Design review of the part built by this model. Coordinates are the model's own, in mm. Face numbers are marked on the shaded views. A direction names the side the tool comes from. Give positions to 0.01 mm unless a question says otherwise; leave off trailing zeros. Order: outer loops, then holes, each group sorted by start corner. A loop starts at its lowest first (then second) coordinate and runs counter-clockwise, first axis right, second up. Notation, with made-up numbers: (68.5, 3) -> (88.5, 3) arc R15 ccw to (88.5, 7) -> close; hole circle Ø4 at (40, 76). An arc over 180 degrees is marked (long way). Return JSON: item names as keys, results as strings.
```python
from build123d import *

# Parameters (mm, degrees)
SKETCH1_W           = 66
SKETCH1_H           = 48
BOSS_EXTRUDE1_DEPTH = 5
SKETCH2_W           = 10
SKETCH2_H           = 10
BOSS_EXTRUDE2_DEPTH = 44
SKETCH3_R           = 1
CUT_EXTRUDE1_DEPTH  = 7
SKETCH4_W           = 66
SKETCH4_H           = 70
BOSS_EXTRUDE3_DEPTH = 3
BOSS_EXTRUDE4_DEPTH = 3
SKETCH6_R           = 1
CUT_EXTRUDE2_DEPTH  = 3


with BuildPart() as part:
    # Sketch1 → Boss-Extrude1 (new body)
    with BuildSketch(Plane(origin=(0, 0, 0), x_dir=(1, 0, 0), z_dir=(0, 1, 0))):
        Rectangle(SKETCH1_W, SKETCH1_H)
    extrude(amount=BOSS_EXTRUDE1_DEPTH)

    # Sketch2 → Boss-Extrude2 (add)
    with BuildSketch(Plane(origin=(0, 5, 0), x_dir=(1, 0, 0), z_dir=(0, 1, 0))):
        with Locations((7, 19)):
            Rectangle(SKETCH2_W, SKETCH2_H)
        with Locations((7, -19)):
            Rectangle(SKETCH2_W, SKETCH2_H)
    extrude(amount=BOSS_EXTRUDE2_DEPTH)

    # Sketch3 → Cut-Extrude1 (cut)
    with BuildSketch(Plane(origin=(0, 49, 0), x_dir=(1, 0, 0), z_dir=(0, 1, 0))):
        with Locations(Location((7, 19, 0), (0, 0, 270))):
            Circle(SKETCH3_R)
        with Locations(Location((7, -19, 0), (0, 0, 270))):
            Circle(SKETCH3_R)
    extrude(amount=-CUT_EXTRUDE1_DEPTH, mode=Mode.SUBTRACT)

    # Sketch4 → Boss-Extrude3 (add)
    with BuildSketch(Plane.XZ):
        Rectangle(SKETCH4_W, SKETCH4_H)
    extrude(amount=BOSS_EXTRUDE3_DEPTH)

    # Sketch5 → Boss-Extrude4 (add)
    with BuildSketch(Plane(origin=(33, 0, 0), x_dir=(0, 0, -1), z_dir=(1, 0, 0))):
        Polygon((-24, 5), (-35, 0), (-24, 0), align=None)
        Polygon((24, 5), (24, 0), (35, 0), align=None)
    boss_extrude4 = extrude(amount=-BOSS_EXTRUDE4_DEPTH)

    # Mirror1: Boss-Extrude4 across plane
    add(boss_extrude4.mirror(Plane(origin=(0, 0, 0), x_dir=(0, 0, 1), z_dir=(1, 0, 0))))

    # Sketch6 → Cut-Extrude2 (cut)
    with BuildSketch(Plane(origin=(0, 0, 0), x_dir=(1, 0, 0), z_dir=(0, 1, 0))):
        with Locations(Location((-22, 29.5, 0), (0, 0, 270))):
            Circle(SKETCH6_R)
        with Locations(Location((22, 29.5, 0), (0, 0, 270))):
            Circle(SKETCH6_R)
    cut_extrude2 = extrude(amount=-CUT_EXTRUDE2_DEPTH, mode=Mode.SUBTRACT)

    # Mirror2: Cut-Extrude2 across plane
    add(cut_extrude2.mirror(Plane.XY), mode=Mode.SUBTRACT)


solid = part.part
```
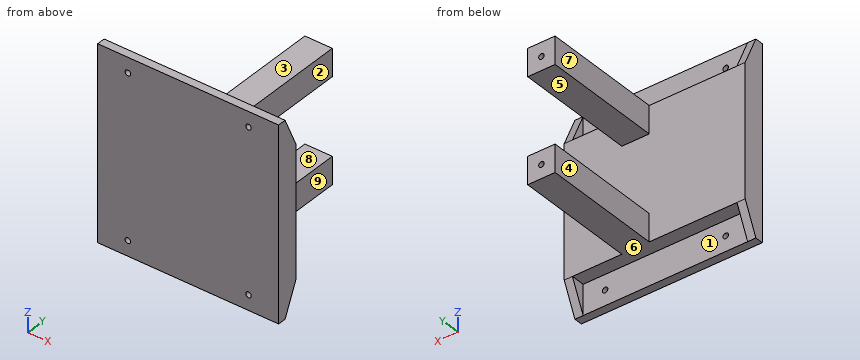
Item 1: Add section B-B (y = 34.5). Give the boundary of the cut face in (x, z), plus the area to 3 significant figures.
Result set:
{"outline": "(2, -24) -> (12, -24) -> (12, -14) -> (2, -14) -> close; (2, 14) -> (12, 14) -> (12, 24) -> (2, 24) -> close", "area": "200 mm^2"}
Item 2: Machinability: for the marked faces 1, 2, 3, 4 and 5, which of the approach directions +Z, -Z, +X, -X, +Y, -Y give a long, thin tool a straight path to every point of the face, cutting with its end or side? Answer none if there is none.
Result set:
{"face 1": "-Z, +Y", "face 2": "+Z, -Z, +X, +Y", "face 3": "+Z, +Y", "face 4": "+Z, -Z, -X, +Y", "face 5": "+X, -X, +Y"}
Item 3: Mouldability with a two-part tool opening along X and no side actions: class the marked faces 6, 7, 8 and 9 as released by +X, released by -X, zero draft, split by the parting line, or undercut.
Result set:
{"face 6": "undercut", "face 7": "released by -X", "face 8": "zero draft", "face 9": "released by +X"}
Item 4: Add section C-C (x = 22). Give the boundary of the cut face in (y, z).
Result set:
{"outline": "(-3, -35) -> (0, -35) -> (0, -30.5) -> (-3, -30.5) -> close; (-3, -28.5) -> (0, -28.5) -> (0, -24) -> (5, -24) -> (5, 24) -> (0, 24) -> (0, 28.5) -> (-3, 28.5) -> close; (-3, 30.5) -> (0, 30.5) -> (0, 35) -> (-3, 35) -> close"}
Item 5: Add section A-A (z = 29.5). Give the boundary of the cut face in (x, y), plus the area to 3 significant figures.
Result set:
{"outline": "(-33, -3) -> (-23, -3) -> (-23, 0) -> (-30, 0) -> (-30, 2.5) -> (-33, 2.5) -> close; (-21, -3) -> (21, -3) -> (21, 0) -> (-21, 0) -> close; (23, -3) -> (33, -3) -> (33, 2.5) -> (30, 2.5) -> (30, 0) -> (23, 0) -> close", "area": "201 mm^2"}
Item 6: For pin 1 (8 mm diameter, centred on x = 5.5, y = 18.5, fed in from +Z); pin 2 (5 mm diameter, centred on y = 27.5, z = 19, fed in from -X); pin 3 (0.6 mm diameter, centred on x = 7, z = 19, fed in from +Y), all flat-tipped, find the tip position at first contact; note any pin that passes through.
Result set:
{"pin 1": "stops at z = 24", "pin 2": "stops at x = 2", "pin 3": "stops at y = 42"}
Item 7: Wall thickness on L1, parallel to X at y = -1.75, z = 29.5; L2, parallel to Z at x = 4.5, y = 44; L3, parallel to Y at x = 18, z = -12.5: over which ranges is each line inside the solid? List them lowest first. Write a range as [from, to].
Result set:
{"L1": "x = [-33, -23], [-21, 21], [23, 33]", "L2": "z = [-24, -14], [14, 24]", "L3": "y = [-3, 5]"}
Item 8: Add section D-D (x = 29). Give the boundary of the cut face in (y, z), plus the area to 3 significant figures.
Result set:
{"outline": "(-3, -35) -> (0, -35) -> (0, -24) -> (5, -24) -> (5, 24) -> (0, 24) -> (0, 35) -> (-3, 35) -> close", "area": "450 mm^2"}
